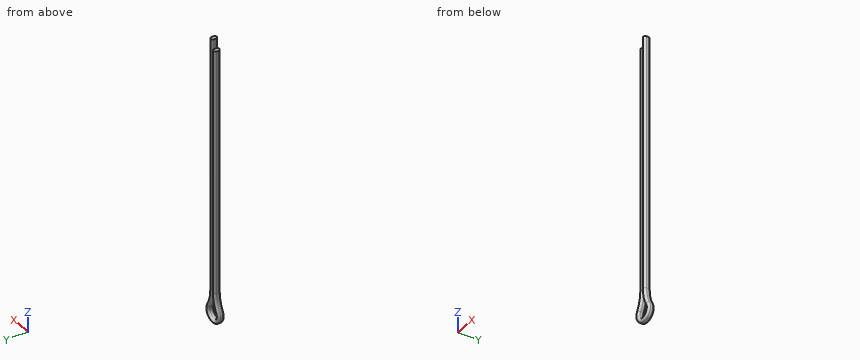
```python
from build123d import *


with BuildPart() as part:
    # Sweep1: sweep along a path in Sketch1
    with BuildLine(Plane(origin=(0, 0, 0), x_dir=(1, 0, 0), z_dir=(0, 1, 0))) as sweep1_path:
        Line((-0.4, 2), (-0.4, 51.5))
        ThreePointArc((-0.4, 51.5), (-0.64900233, 53.359363001), (-1.378461538, 55.087692308))
        ThreePointArc((-1.378461538, 55.087692308), (0, 57.5), (1.378461538, 55.087692308))
        ThreePointArc((1.378461538, 55.087692308), (0.64900233, 53.359363001), (0.4, 51.5))
        Line((0.4, 51.5), (0.4, 0))
    # Sketch2 → Sweep1 (sweep)
    with BuildSketch(Plane.XY):
        with BuildLine():
            Line((0, -0.2), (0, 0.2))
            ThreePointArc((0, 0.2), (0.4, 0.6), (0.8, 0.2))
            Line((0.8, 0.2), (0.8, -0.2))
            ThreePointArc((0.8, -0.2), (0.4, -0.6), (0, -0.2))
        make_face()
    sweep(path=sweep1_path.line)


solid = part.part
```
Read the model definition and answer for the solid it produces. Units are mm, in the model's axes. Give positions to 0.01 mm unless a question says otherwise; leave off trailing zeros. Order: outer loops, then holes, each group sorted by start corner. A loop starts at its lowest first (then second) coordinate and runs counter-clockwise, first axis right, second up.
(1) A straight line is drawn through the part: L1, parallel to X at y = 0.15, z = -55.9. Find the intervals that lie inside material, in ascending order.
(2) Find section B-B (y = 0.4). Give the vertices of the cut face in (x, z).
(3) Given pin 1 (0.6 mm diameter, centred on x = -0.5, y = 0, fed in from +Z); pin 2 (1 mm diameter, centred on x = 1, z = -43.5, fed in from -Y), each flat-ended and moving along its own axis, determine where each tip first touches the part or whether it passes through.
(4) Find section A-A (z = -49.5). Give the vertices of the cut face in (x, y).
Result sheet:
1. L1: x = -2 to -1.2, 1.2 to 2
2. outline: (-1.68, -54.91) arc R1.95 ccw (long way) to (1.68, -54.91) arc R6.72 cw to (0.75, -51.5) - (0.75, 0) - (0.05, 0) - (0.05, -51.5) arc R7.41 ccw to (1.08, -55.26) arc R1.25 cw (long way) to (-1.08, -55.26) arc R7.41 ccw to (-0.05, -51.5) - (-0.05, -2) - (-0.75, -2) - (-0.75, -51.5) arc R6.72 cw to start
3. pin 1: stops at z = -2
3. pin 2: stops at y = -0.59
4. outline: (-0.8, -0.2) arc R0.4 ccw to (0, -0.2) arc R0.4 ccw to (0.8, -0.2) - (0.8, 0.2) arc R0.4 ccw to (0, 0.2) arc R0.4 ccw to (-0.8, 0.2) - close
